Could you check a few things on this model? Use its own coordinates, in mm. A direction names the side the tool comes from. Give positions to 0.01 mm unless a question says otherwise; leave off trailing zeros. Order: outer loops, then holes, each group sorted by start corner. A loop starts at its lowest first (then second) coordinate and runs counter-clockwise, first axis right, second up. Notation, with made-up numbers: M 41.5,30 L 60.5,30 A21 ccw 60.5,58 Z; hole C -22.5,-36 d5. An arc over 180 degrees is marked long. Use a Markdown table: item, result. Add a question column.
Item 1: If we mould it in two halves opening along Y, with no side actions, what happens to faces 1 (the face through (-9.945, 9.12, 6.261)), 2 (the face through (-12, -2, 12.7)), 3 (the face through (11.99, 0.53, 1.96))? For each: released by +Y, released by -Y, zero draft, split by the parting line, or undercut.
Item 2: Suppose I cut it at C-C on z = 5.25. Write out the boundary of the cut face in (x, y), plus the area to 3 significant figures.
Item 3: If I drill on L1, parallel to Y at x = 0, z = 5; L2, parallel to Y at x = 0, z = 2.05; L3, parallel to Z at x = 6.5, y = 6.5, over which ranges is the centre line in solid material (lowest first)? Write a range as from..to.
Item 4: Suppose I cut it at A-A on x = 0. Write out the boundary of the cut face in (y, z).
Item 5: For faces 4 (the face through (-12, -2, 0)), 5 (the face through (5, -8, 3.969)), 6 (the face through (5, -8, 6.191)), which set-ups out of +Z, -Z, +X, -X, +Y, -Y let a thin tool reach every point of the face, with its end or its side?
Item 6: Suppose I cut it at D-D on z = 1.5. Write out the boundary of the cut face in (x, y), plus the area to 3 significant figures.
Item 7: I'm going to push flat-ended pins straight in: pin 1 Ø4 at (x, z) = (5, 8.5) entering from -Y; pin 2 Ø7 at (x, y) = (-4, 4) entering from -Z; pin 3 Ø6 at (y, z) = (-1, 10.5) entering from +X; pin 4 Ø1 at (x, y) = (-5, 7) entering from +Z. Where does each tip first touch, or does it pass through?
from build123d import *

# Parameters (mm, degrees)
SKETCH1_R           = 13.49375
BOSS_EXTRUDE1_DEPTH = 12.7
SKETCH3_R           = 12
CUT_EXTRUDE2_DEPTH  = 23.922752412
SKETCH4_R           = 12
BOSS_EXTRUDE2_DEPTH = 2.2225
SKETCH5_R           = 8.95
CUT_EXTRUDE3_DEPTH  = 21.162499961


with BuildPart() as part:
    # Sketch1 → Boss-Extrude1 (new body)
    with BuildSketch(Plane.XY):
        Circle(SKETCH1_R)
    extrude(amount=BOSS_EXTRUDE1_DEPTH)

    # Sketch3 → Cut-Extrude2 (cut, through all)
    with BuildSketch(Plane(origin=(0, 0, 0), x_dir=(-1, 0, 0), z_dir=(0, 0, -1))):
        Circle(SKETCH3_R)
    extrude(amount=-CUT_EXTRUDE2_DEPTH, mode=Mode.SUBTRACT)

    # Sketch4 → Boss-Extrude2 (add)
    with BuildSketch(Plane(origin=(0, 0, 3.96875), x_dir=(-1, 0, 0), z_dir=(0, 0, -1))):
        Circle(SKETCH4_R)
    extrude(amount=-BOSS_EXTRUDE2_DEPTH)

    # Sketch5 → Cut-Extrude3 (cut, through all)
    with BuildSketch(Plane.XY.offset(6.19125)):
        Circle(SKETCH5_R)
    extrude(amount=-CUT_EXTRUDE3_DEPTH, mode=Mode.SUBTRACT)


solid = part.part
Findings below:
| question | item | result |
|---|---|---|
| 1 | face 1 | split by the parting line |
| 1 | face 2 | zero draft |
| 1 | face 3 | undercut |
| 2 | outline | C 0,0 d26.99; hole C 0,0 d17.9 |
| 2 | area | 320 mm^2 |
| 3 | L1 | y = -13.49..-8.95, 8.95..13.49 |
| 3 | L2 | y = -13.49..-12, 12..13.49 |
| 3 | L3 | z = 3.97..6.19 |
| 4 | outline | M -13.49,0 L -12,0 L -12,3.97 L -8.95,3.97 L -8.95,6.19 L -12,6.19 L -12,12.7 L -13.49,12.7 Z; M 8.95,3.97 L 12,3.97 L 12,0 L 13.49,0 L 13.49,12.7 L 12,12.7 L 12,6.19 L 8.95,6.19 Z |
| 5 | face 4 | -Z, +X, -X, +Y, -Y |
| 5 | face 5 | -Z |
| 5 | face 6 | +Z |
| 6 | outline | C 0,0 d26.99; hole C 0,0 d24 |
| 6 | area | 120 mm^2 |
| 7 | pin 1 | stops at y = -13.16 |
| 7 | pin 2 | stops at z = 3.97 |
| 7 | pin 3 | stops at x = 13.49 |
| 7 | pin 4 | stops at z = 6.19 |
